Check sheet for the drawn part. Datum: minimum x, y, z corner. Units: mm. Give positions to 0.01 mm unless a question says otherwise; leave off trailing zeros. Write each loop counter-clockwise with the first axis right and the second up, starting at its lowest first coordinate (ties: lowest second). Pieces come first, ordered by that corner, then holes. Notation, with made-up numbers: (31.25, 24) -> (50.25, 24) arc R15 cw to (50.25, 36) -> close; hole circle Ø7 at (47, 32). An arc over 180 degrees is marked (long way). Answer as CSV lines item,"result". Start each with the question number.
1) Sectioned sample at D-D on z = 45.5. Record the cut outline in (x, y).
2) Sectioned sample at B-B on z = 140. Record the cut outline in (x, y), and give its area (3 significant figures).
3) Material ranges on L1, parallel to X at y = 69, z = 20.5; L2, parallel to Y at x = 105.5, z = 165.5; L3, parallel to X at y = 118, z = 170.5, recorded low to high.
4) Sectioned sample at C-C on y = 39. Record the cut outline in (x, z).
5) Sectioned sample at A-A on y = 15. Record the cut outline in (x, z).
6) Gauge pin test, flat ends, axial feed: pin 1 Ø5 at (x, z) = (139, 187) entering from -Y; pin 2 Ø7.5 at (x, z) = (39.072, 190.953) entering from -Y; pin 3 Ø4 at (x, z) = (39.072, 102.741) entering from +Y; pin 4 Ø3 at (x, y) = (6.5, 56.5) entering from +Z. Record the tip position at first contact, or that the pin passes through.
7) Mould release check, pull along X, two halves, no side actions. Record for the marked faces 1, 2, 3 and 4: released by +X, released by -X, zero draft, split by the parting line, or undercut.
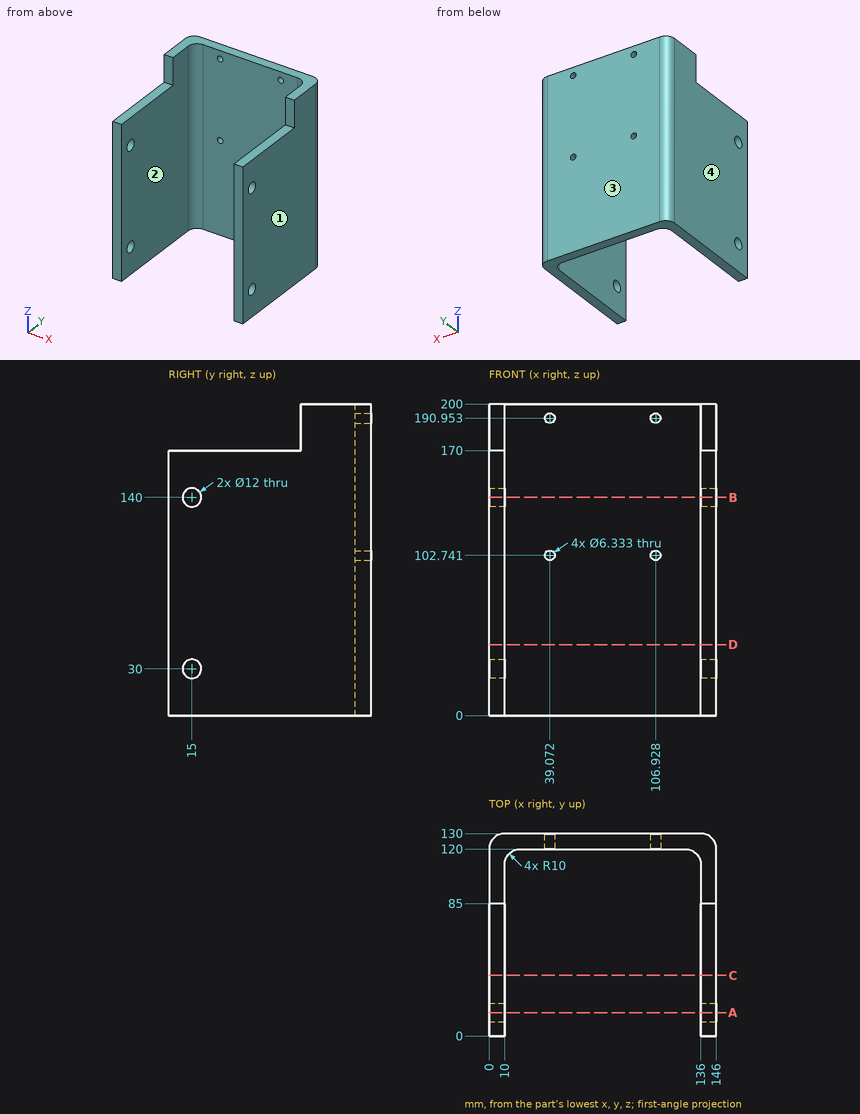
Ans:
1,outline,"(0, 0) -> (10, 0) -> (10, 110) arc R10 cw to (20, 120) -> (126, 120) arc R10 cw to (136, 110) -> (136, 0) -> (146, 0) -> (146, 120) arc R10 ccw to (136, 130) -> (10, 130) arc R10 ccw to (0, 120) -> close"
2,outline,"(0, 0) -> (10, 0) -> (10, 9) -> (0, 9) -> close; (0, 21) -> (10, 21) -> (10, 110) arc R10 cw to (20, 120) -> (126, 120) arc R10 cw to (136, 110) -> (136, 21) -> (146, 21) -> (146, 120) arc R10 ccw to (136, 130) -> (10, 130) arc R10 ccw to (0, 120) -> close; (136, 0) -> (146, 0) -> (146, 9) -> (136, 9) -> close"
2,area,"3,620 mm²"
3,L1,"x = 0 to 10, 136 to 146"
3,L2,"y = 120 to 130"
3,L3,"x = 0 to 14, 132 to 146"
4,outline,"(0, 0) -> (10, 0) -> (10, 170) -> (0, 170) -> close; (136, 0) -> (146, 0) -> (146, 170) -> (136, 170) -> close"
5,outline,"(0, 0) -> (10, 0) -> (10, 24) -> (0, 24) -> close; (0, 36) -> (10, 36) -> (10, 134) -> (0, 134) -> close; (0, 146) -> (10, 146) -> (10, 170) -> (0, 170) -> close; (136, 0) -> (146, 0) -> (146, 24) -> (136, 24) -> close; (136, 36) -> (146, 36) -> (146, 134) -> (136, 134) -> close; (136, 146) -> (146, 146) -> (146, 170) -> (136, 170) -> close"
6,pin 1,"stops at y = 85"
6,pin 2,"stops at y = 120"
6,pin 3,"passes through"
6,pin 4,"stops at z = 170"
7,face 1,"released by +X"
7,face 2,"undercut"
7,face 3,"zero draft"
7,face 4,"released by -X"
